from build123d import *

# Parameters (mm, degrees)
ESQUISSE3_R             = 35
BOSS_EXTRU_3_DEPTH      = 5
ESQUISSE5_R             = 1.5
ENL_V_MAT_EXTRU_1_DEPTH = 161.669919512
ESQUISSE7_R             = 2
ENL_V_MAT_EXTRU_2_DEPTH = 10


with BuildPart() as part:
    # Esquisse3 → Boss.-Extru.3 (new body)
    with BuildSketch(Plane(origin=(0, 0, 0), x_dir=(1, 0, 0), z_dir=(0, 1, 0))):
        with BuildLine():
            Line((-115, -25), (-25, -25))
            Line((-25, -25), (-24.99494949, -24.500051021))
            ThreePointArc((-24.99494949, -24.500051021), (-34.998214236, 0.353553761), (-24.494897428, 25))
            Line((-24.494897428, 25), (-25, 25))
            Line((-25, 25), (-115, 25))
            Line((-115, 25), (-115, -25))
        make_face()
        Circle(ESQUISSE3_R)
        Polygon((-9.403186381, -33.713203436), (35.849364905, -112.092921435), (79.150635095, -87.092921435), (34.150635095, -9.150635095), align=None)
        with BuildLine():
            Line((-24.494897428, 25), (-24.99494949, -24.500051021))
            ThreePointArc((-24.99494949, -24.500051021), (-17.805293657, -30.132565736), (-9.403186381, -33.713203436))
            Line((-9.403186381, -33.713203436), (33.715141323, -9.396235714))
            ThreePointArc((33.715141323, -9.396235714), (34.677297662, -4.741837919), (35, 0))
            ThreePointArc((35, 0), (34.72342821, 4.391302011), (33.898083809, 8.713203436))
            Line((33.898083809, 8.713203436), (-8.720191833, 33.896286735))
            ThreePointArc((-8.720191833, 33.896286735), (-17.19292058, 30.486119496), (-24.494897428, 25))
        make_face()
        Circle(ESQUISSE3_R)
        Polygon((33.898083809, 8.713203436), (79.150635095, 87.092921435), (35.849364905, 112.092921435), (-9.150635095, 34.150635095), align=None)
        with BuildLine():
            ThreePointArc((33.898083809, 8.713203436), (17.805293657, 30.132565736), (-8.720191833, 33.896286735))
            Line((-8.720191833, 33.896286735), (33.898083809, 8.713203436))
        make_face()
    extrude(amount=BOSS_EXTRU_3_DEPTH)

    # Esquisse5 → Enlèv. mat.-Extru.1 (cut, through all)
    with BuildSketch(Plane(origin=(0, 5, 0), x_dir=(1, 0, 0), z_dir=(0, 1, 0))):
        with BuildLine():
            Line((30.514428415, 97.852540378), (20.514428415, 80.532032303))
            ThreePointArc((20.514428415, 80.532032303), (21.429491924, 77.116968793), (24.844555434, 78.032032303))
            Line((24.844555434, 78.032032303), (34.844555434, 95.352540378))
            ThreePointArc((34.844555434, 95.352540378), (33.929491924, 98.767603888), (30.514428415, 97.852540378))
        make_face()
        with BuildLine():
            ThreePointArc((10.514428415, 63.211524227), (13.929491924, 64.126587737), (14.844555434, 60.711524227))
            Line((14.844555434, 60.711524227), (4.844555434, 43.391016151))
            ThreePointArc((4.844555434, 43.391016151), (1.429491924, 42.475952642), (0.514428415, 45.891016151))
            Line((0.514428415, 45.891016151), (10.514428415, 63.211524227))
        make_face()
        with BuildLine():
            ThreePointArc((65.155444566, 77.852540378), (68.570508076, 78.767603888), (69.485571585, 75.352540378))
            Line((69.485571585, 75.352540378), (59.485571585, 58.032032303))
            ThreePointArc((59.485571585, 58.032032303), (56.070508076, 57.116968793), (55.155444566, 60.532032303))
            Line((55.155444566, 60.532032303), (65.155444566, 77.852540378))
        make_face()
        with BuildLine():
            Line((45.155444566, 43.211524227), (35.155444566, 25.891016151))
            ThreePointArc((35.155444566, 25.891016151), (36.070508076, 22.475952642), (39.485571585, 23.391016151))
            Line((39.485571585, 23.391016151), (49.485571585, 40.711524227))
            ThreePointArc((49.485571585, 40.711524227), (48.570508076, 44.126587737), (45.155444566, 43.211524227))
        make_face()
        with Locations(Location((35, -60.621778265, 0), (0, 0, 270))):
            Circle(ESQUISSE5_R)
        with Locations(Location((-70, 0, 0), (0, 0, 270))):
            Circle(ESQUISSE5_R)
    extrude(amount=-ENL_V_MAT_EXTRU_1_DEPTH, mode=Mode.SUBTRACT)

    # Esquisse7 → Enlèv. mat.-Extru.2 (cut)
    with BuildSketch(Plane(origin=(0, 5, 0), x_dir=(1, 0, 0), z_dir=(0, 1, 0))):
        with Locations(Location((69.722431864, 86.762794416, 0), (0, 0, 270))):
            Circle(ESQUISSE7_R)
        with Locations(Location((-109.562568341, -17.757653858, 0), (0, 0, 270))):
            Circle(ESQUISSE7_R)
        with Locations(Location((68.847568546, -86.762794416, 0), (0, 0, 270))):
            Circle(ESQUISSE7_R)
    extrude(amount=-ENL_V_MAT_EXTRU_2_DEPTH, mode=Mode.SUBTRACT)


solid = part.part
Can you work these out from the model? Positions are in its coordinate system, mm. A direction names the side the tool comes from. Give positions to 0.01 mm unless a question says otherwise; leave off trailing zeros. Loops run counter-clockwise (first coordinate to the right, second up) from the corner with the lowest first, then second, coordinate; pieces in that order, holes last. Notation, with made-up numbers: (9, -6) -> (21, -6) arc R28 cw to (21, 25) -> close; hole circle Ø4 at (82, 19). An arc over 180 degrees is marked (long way). Write item = value, one per line.
1) Will these pins go through, and if not, where does the flat tip stop? pin 1 (2.5 mm diameter, centred on x = 69.72, z = -86.76, fed in from +Y); pin 2 (1.5 mm diameter, centred on x = -45, y = 4.5, fed in from -Z); pin 3 (2.5 mm diameter, centred on x = -81.5, y = 3, fed in from +Z).
Check result:
pin_1 = through
pin_2 = -25
pin_3 = 25
2) For faces 4 (the flat face through (56.966, 2.465, 48.667)), 5 (the flat face through (40.225, 2.535, -34.673)), 6 (the flat face through (12.906, 2.465, 72.354)), which set-ups out of +Z, -Z, +X, -X, +Y, -Y let a thin tool reach every point of the face, with its end or its side?
Check result:
face_4 = +X, +Y, -Y
face_5 = +Y, -Y
face_6 = +Z, -X, +Y, -Y
3) I need wall thicknesses on L1, parallel to X at y = 1.45, z = 0; L2, parallel to Z at x = 62.5, y = 4.8; L3, parallel to Z at x = 65, y = 4.35. Which ranges of each line are inside material? Lowest first, please. Write a range as from..to.
Check result:
L1 = -115..-71.5, -68.5..35
L2 = -96.71..-73.25, -63.25..-58.25, 58.25..96.71
L3 = -95.26..-77.58, -67.58..-62.58, 62.58..95.26
4) Suppose I cut it at B-B on x = -80. Write out the boundary of the cut face in (y, z), then the cut area to 3 significant figures.
Check result:
outline = (0, -25) -> (5, -25) -> (5, 25) -> (0, 25) -> close
area = 250 mm2
5) Suppose I cut it at A-A on z = -54. Write out the boundary of the cut face in (x, y).
Check result:
outline = (2.31, 0) -> (5.2, 0) -> (5.2, 5) -> (2.31, 5) -> close; (10.97, 0) -> (60.04, 0) -> (60.04, 5) -> (10.97, 5) -> close
6) Thinking about a two-plate mould opening in X: for faces 1 (the flat face through (56.208, 2.465, -47.354)), 2 (the cylindrical face through (68.523, 2.535, -78.795)), 3 (the flat face through (-71, 2, 25)), which applies, released by +X, released by -X, zero draft, split by the parting line, or undercut?
Check result:
face_1 = released by +X
face_2 = undercut
face_3 = zero draft
7) Suppose I cut it at C-C on y = 2.2. Give the number of separate pieces and of enclosed holes in the cut face, then the cut area to 3 significant figures.
Check result:
separate_pieces = 1
enclosed_holes = 9
area = 15,800 mm2
